Check sheet for the drawn part. Datum: minimum x, y, z corner. Units: mm. A direction names the side the tool comes from. Coordinates: 2 decimals unless noted, no trailing zeros. Loops run counter-clockwise (first coordinate to the right, second up) from the corner with the lowest first, then second, coordinate; pieces in that order, holes last.
Q1. Material ranges on probe 1 along X at (y, z) = (11, 14.25); probe 2 along Y at (x, z) = (7, 16); probe 3 along Z at (x, y) = (10.5, 16.25), recorded low to high.
Q2. Access from +Z, -Z, +X, -X, +Y, -Y to the whole of each face (thin tool, end or side, straight path). Record for the marked faces 4 and 5.
Q3. Sectioned sample at B-B (z = 8). Enter the section's corners in (x, y).
Q4. Sectioned sample at D-D (y = 3). Enter the section's corners in (x, z), then the cut area to 3 significant figures.
Q5. Sectioned sample at A-A (x = 8.5). Enter the section's corners in (y, z), then the cut area to 3 significant figures.
Q6. Mould release check, pull along X, two halves, no side actions. Record for the marked faces 1, 2 and 3: +X half, -X half, draft (parallel to the pull), parting line (faces both ways), or undercut.
Q7. Sectioned sample at C-C (y = 9). Enter the section's corners in (x, z).
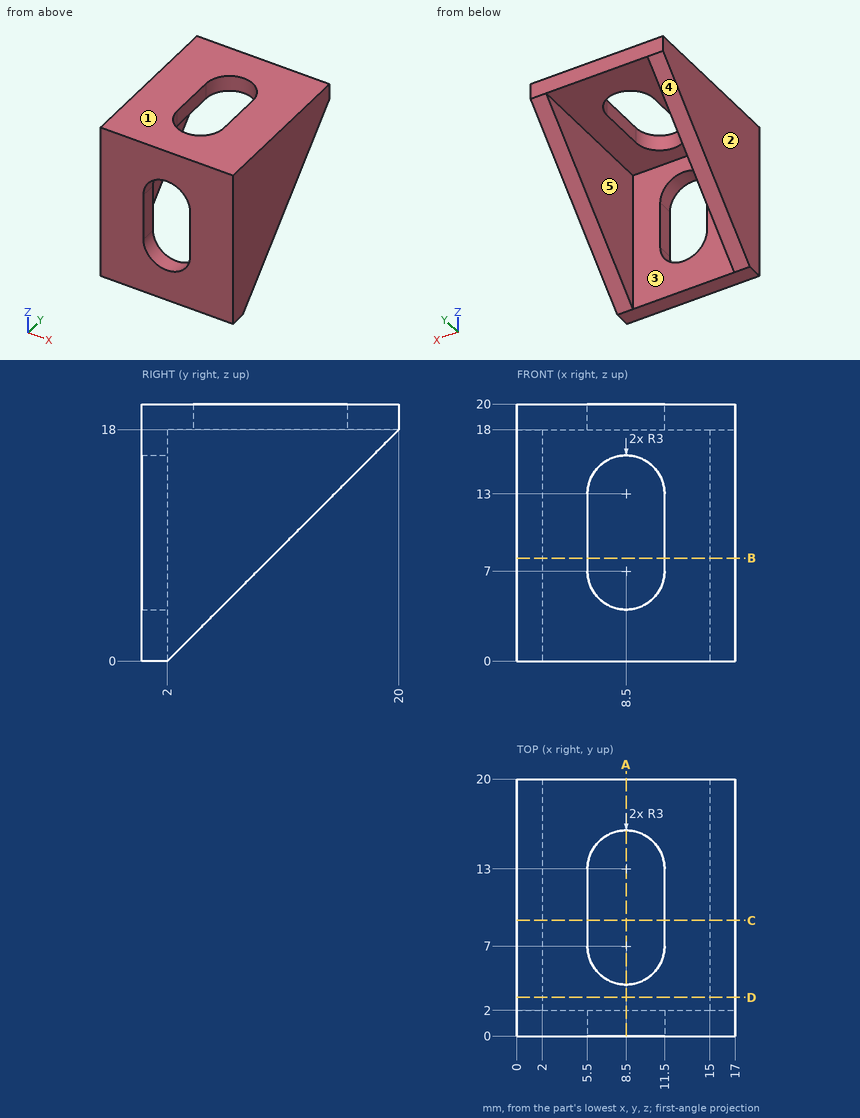
Geometry check:
1. probe 1: x = 0 to 2, 15 to 17
1. probe 2: y = 0 to 2
1. probe 3: z = 18 to 20
2. face 4: -Z, +X, -X, +Y
2. face 5: -Z, +Y
3. outline: (0, 0) - (5.5, 0) - (5.5, 2) - (2, 2) - (2, 10) - (0, 10) - close; (11.5, 0) - (17, 0) - (17, 10) - (15, 10) - (15, 2) - (11.5, 2) - close
4. outline: (0, 1) - (2, 1) - (2, 18) - (15, 18) - (15, 1) - (17, 1) - (17, 20) - (0, 20) - close
4. area: 102 mm2
5. outline: (0, 0) - (2, 0) - (2, 4) - (0, 4) - close; (0, 16) - (2, 16) - (2, 18) - (4, 18) - (4, 20) - (0, 20) - close; (16, 18) - (20, 18) - (20, 20) - (16, 20) - close
5. area: 28.0 mm2
6. face 1: draft
6. face 2: -X half
6. face 3: undercut
7. outline: (0, 7) - (2, 7) - (2, 18) - (5.5, 18) - (5.5, 20) - (0, 20) - close; (11.5, 18) - (15, 18) - (15, 7) - (17, 7) - (17, 20) - (11.5, 20) - close
